```python
from build123d import *

# Parameters (mm, degrees)
F1_DEPTH = 48
F2_R     = 5
F3_DEPTH = 11.001
F5_DEPTH = 15.748
F6_R     = 2.5
F7_DEPTH = 41.001
F8_R     = 1.064771
F9_R     = 5


with BuildPart() as f1:
    # F0 (on Front) → F1 (new body)
    with BuildSketch(Plane.XZ):
        with BuildLine():
            Line((-27.910571, 11), (-56, 11))
            Line((-56, 11), (-56, 0))
            Line((-56, 0), (-19, 0))
            ThreePointArc((-19, 0), (0, 19), (19, 0))
            Line((19, 0), (51, 0))
            Line((51, 0), (51, 41))
            Line((51, 41), (40, 41))
            Line((40, 41), (40, 11))
            Line((40, 11), (27.910571, 11))
            ThreePointArc((27.910571, 11), (0, 30), (-27.910571, 11))
        make_face()
    extrude(amount=-F1_DEPTH)

    # F2 (on face) → F3 (cut, through all)
    with BuildSketch(Plane.XY.offset(11)):
        with Locations((-43, 35)):
            Circle(F2_R)
        with Locations((-43, 13)):
            Circle(F2_R)
        with BuildLine():
            Line((-56, 48), (-56, 35))
            ThreePointArc((-56, 35), (-52.192388, 44.192388), (-43, 48))
            Line((-43, 48), (-56, 48))
        make_face()
        with BuildLine():
            Line((-56, 0), (-43, 0))
            ThreePointArc((-43, 0), (-52.192388, 3.807612), (-56, 13))
            Line((-56, 13), (-56, 0))
        make_face()
    extrude(amount=-F3_DEPTH, mode=Mode.SUBTRACT)

    # F4 (on face) → F5 (cut)
    with BuildSketch(Plane.YZ.offset(51)):
        with BuildLine():
            Line((30.5, 41), (17.5, 41))
            Line((17.5, 41), (17.5, 25))
            ThreePointArc((17.5, 25), (24, 18.5), (30.5, 25))
            Line((30.5, 25), (30.5, 41))
        make_face()
    extrude(amount=-F5_DEPTH, mode=Mode.SUBTRACT)

    # F6 (on face) → F7 (cut, through all)
    with BuildSketch(Plane(origin=(0, 0, 0), x_dir=(1, 0, 0), z_dir=(0, 0, -1))):
        with Locations((0, -24)):
            Circle(F6_R)
    extrude(amount=-F7_DEPTH, mode=Mode.SUBTRACT)

    # F8
    f8_edges = [f1.edges().sort_by_distance(p)[0] for p in [
        (-2.5, 24, 29.895652),
    ]]
    fillet(f8_edges, radius=F8_R)

    # F9
    f9_edges = [f1.edges().sort_by_distance(p)[0] for p in [
        (45.5, 0, 41),
        (45.5, 48, 41),
    ]]
    fillet(f9_edges, radius=F9_R)


solid = f1.part
```
Here's how the part is built. I have some questions about the finished solid (model axes, mm). A direction names the side the tool comes from. Round coordinates to 2 decimals unless told otherwise and drop trailing zeros. Order: outer loops, then holes, each group sorted by start corner. A loop starts at its lowest first (then second) coordinate and runs counter-clockwise, first axis right, second up. Notation, with made-up numbers: M -35,82.5 L -15,82.5 A19 ccw -15,101.5 Z; hole C 31,81 d3. An arc over 180 degrees is marked long. Answer in a Markdown table with one row per item.
Item 1: Imagine slicing it at D-D, the plane x = 15.5. Write out the boundary of the cut face in (y, z).
A:
| item | result |
|---|---|
| outline | M 0,10.99 L 48,10.99 L 48,25.69 L 0,25.69 Z |
Item 2: Thinking about a two-plate mould opening in Y: for faces 4 (the face through (-38, 24, 0)), 5 (the face through (46, 30.5, 33)), 6 (the face through (14, 48, 14)), 7 (the face through (14, 0, 14)), which applies, +Y half, -Y half, draft (parallel to the pull), parting line (faces both ways), or undercut?
A:
| item | result |
|---|---|
| face 4 | draft |
| face 5 | undercut |
| face 6 | +Y half |
| face 7 | -Y half |
Item 3: I'm going to push flat-ended pins straight in: pin 1 (8 mm diameter, centred on x = -43, y = 35, fed in from +Z); pin 2 (4 mm diameter, centred on x = -1, y = 35, fed in from -Z); pin 3 (12 mm diameter, centred on x = 5.5, y = 7, fed in from -Z); pin 4 (3 mm diameter, centred on y = 8, z = 15.5, fed in from -X). Where does each tip first touch, or does it pass through?
A:
| item | result |
|---|---|
| pin 1 | passes through |
| pin 2 | stops at z = 18.76 |
| pin 3 | stops at z = 15.12 |
| pin 4 | stops at x = -26.53 |
Item 4: Imagine slicing it at B-B, the plane x = -39. Write out the boundary of the cut face in (y, z).
A:
| item | result |
|---|---|
| outline | M 0,0 L 10,0 L 10,11 L 0,11 Z; M 16,0 L 32,0 L 32,11 L 16,11 Z; M 38,0 L 48,0 L 48,11 L 38,11 Z |
Item 5: If I drill on L1, parallel to Y at x = -43, z = 4.75; L2, parallel to X at y = 8.5, z = 6.5; L3, parallel to Z at x = -44.5, y = 44.5, over which ranges is the centre line in solid material (lowest first)? Write a range as from..to.
A:
| item | result |
|---|---|
| L1 | y = 0..8, 18..30, 40..48 |
| L2 | x = -55.2..-45.18, -40.82..-17.85, 17.85..51 |
| L3 | z = 0..11 |
Item 6: Imagine slicing it at C-C, the plane z = 34. Write out the boundary of the cut face in (x, y).
A:
| item | result |
|---|---|
| outline | M 40,0 L 51,0 L 51,17.5 L 40,17.5 Z; M 40,30.5 L 51,30.5 L 51,48 L 40,48 Z |
Item 7: Imagine slicing it at A-A, the plane z = 7.5. Write out the boundary of the cut face in (x, y).
A:
| item | result |
|---|---|
| outline | M -56,13 A13 ccw -43,0 L -17.46,0 L -17.46,48 L -43,48 A13 ccw -56,35 Z; M 17.46,0 L 51,0 L 51,48 L 17.46,48 Z; hole C -43,13 d10; hole C -43,35 d10 |
Item 8: For faces 1 (the face through (46, 17.5, 33)), 2 (the face through (6.104, 23.664, 17.993)), 3 (the face through (-42, 24, 11)), which set-ups out of +Z, -Z, +X, -X, +Y, -Y let a thin tool reach every point of the face, with its end or its side?
A:
| item | result |
|---|---|
| face 1 | +Z, +X |
| face 2 | -Z, +Y, -Y |
| face 3 | +Z, -X, +Y, -Y |
